For this review, take the finished solid that the model builds, in its own axes (mm). A direction names the side the tool comes from. Round coordinates to 2 decimals unless told otherwise and drop trailing zeros. Loops run counter-clockwise (first coordinate to the right, second up) from the corner with the lowest first, then second, coordinate; pieces in that order, holes last.
```python
from build123d import *


with BuildPart() as part:
    # Sketch1 → Revolve1 (revolve)
    with BuildSketch(Plane.XY, mode=Mode.PRIVATE) as revolve1_sk:
        Polygon((0, 0), (0, 1.5), (-1.5, 5), (-1.5, 6.25), (1.5, 6.25), (1.5, 3.5), (13.5, 3.5), (15, 2), (20.875, 2), (21, 1.875), (21, 1), (24, 1), (24, 1.875), (24.125, 2), (30, 2), (31, 1), (31, 0), align=None)
    revolve(revolve1_sk.sketch.rotate(Axis((31, 0, 0), (-1, 0, 0)), 90), axis=Axis((31, 0, 0), (-1, 0, 0)))


solid = part.part
```
(1) Insertion check: pin 1 Ø4 at (x, z) = (8.5, -4) entering from -Y; pin 2 Ø2 at (y, z) = (-4.5, -4) entering from +X; pin 3 Ø5 at (y, z) = (2.5, 3.5) entering from +X. Each pin has a flat end and moves straight along its axis. Give the tip position at first contact, or say it passes through.
(2) Add section C-C (x = 13). Give the boundary of the cut face in (y, z), plus the area to 3 significant figures.
(3) For faces 1 (the cylindrical face through (18, 2, 0)), 2 (the cylindrical face through (0.02, -1.88, -5.96)), 3 (the cylindrical face through (23, 1, 0)), list the 3-axis set-ups (+Z, -Z, +X, -X, +Y, -Y) from which the entire face can be reached by the end or side of a thin tool; tool diameter is ignored.
(4) The part is to be moulded in two halves that separate along Z. For faces 4 (the flat face through (1.5, 3, -3)), 5 (the flat face through (0, 0, 0)), 6 (the cylindrical face through (7.584, 3.105, -1.615)), say which applies: pulls with the +Z half, pulls with the -Z half, needs draft (parallel to the pull), parting line crosses it, or undercut.
(5) Add section D-D (x = 20). Give the boundary of the cut face in (y, z).
(6) For L1, parallel to X at y = 4.75, z = -2; L2, parallel to Z at x = 15, y = -0.5; L3, parallel to Z at x = 8, y = -2.5, list the stretches that pass through material, from the lowest coordinate up.
Outcome:
1. pin 1: stops at y = -2.87
1. pin 2: stops at x = 1.5
1. pin 3: stops at x = 30.2
2. outline: circle Ø7 at (0, 0)
2. area: 38.5 mm2
3. face 1: +X
3. face 2: +X, -X
3. face 3: none
4. face 4: needs draft
4. face 5: undercut
4. face 6: parting line crosses it
5. outline: circle Ø4 at (0, 0)
6. L1: x = -1.5 to 1.5
6. L2: z = -1.94 to 1.94
6. L3: z = -2.45 to 2.45
